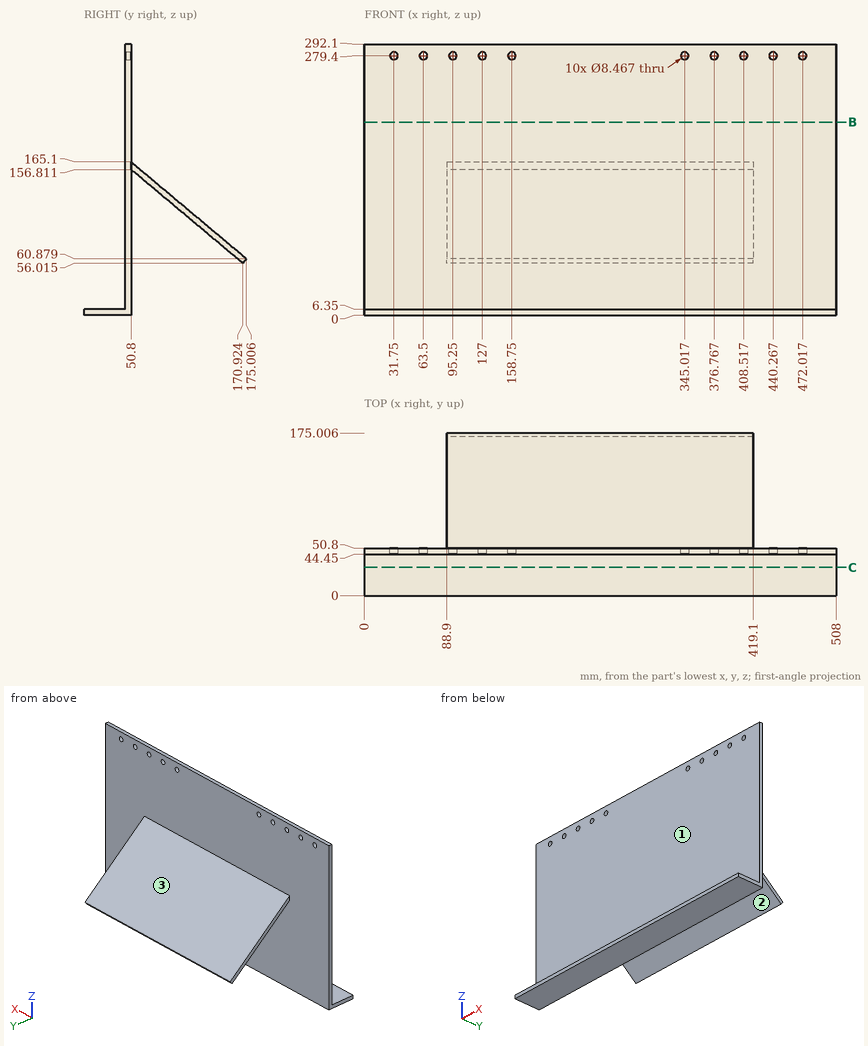
Print and shaded views of the part. All mm, measured from the part's lowest x, y and z. Coordinates: 2 decimals unless noted, no trailing zeros. Order: outer loops, then holes, each group sorted by start corner. A loop starts at its lowest first (then second) coordinate and runs counter-clockwise, first axis right, second up.
Item 1: Drop flat-ended pins along their axis: pin 1 Ø11 at (x, z) = (127, 279.4) entering from -Y; pin 2 Ø5 at (x, y) = (363, 76) entering from -Z; pin 3 Ø13.5 at (x, z) = (440.27, 279.4) entering from +Y. Give the stop position or say it passes through.
Filled in:
pin 1: stops at y = 44.45
pin 2: stops at z = 133.57
pin 3: stops at y = 50.8
Item 2: Drill centre lines: L1, parallel to Z at x = 63.5, y = 48; L2, parallel to Y at x = 242, z = 248; L3, parallel to Z at x = 444.5, y = 10. Where is each one in solid material? Low to high.
Filled in:
L1: z = 0 to 275.17, 283.63 to 292.1
L2: y = 44.45 to 50.8
L3: z = 0 to 6.35
Item 3: Mould opens along Y. For the marked faces 1, 2 and 3 say: released by +Y, released by -Y, zero draft, split by the parting line, or undercut.
Filled in:
face 1: released by -Y
face 2: undercut
face 3: released by +Y
Item 4: Saw through at C-C on y = 30.5. List the corners of the cut face in (x, z).
Filled in:
outline: (0, 0) - (508, 0) - (508, 6.35) - (0, 6.35) - close
Item 5: Saw through at B-B on z = 208. List the corners of the cut face in (x, y), then the cut area to 3 significant figures.
Filled in:
outline: (0, 44.45) - (508, 44.45) - (508, 50.8) - (0, 50.8) - close
area: 3,230 mm2
